```python
from build123d import *

# Parameters (mm, degrees)
SKETCH1_W           = 25
SKETCH1_H           = 21
BOSS_EXTRUDE1_DEPTH = 5
BOSS_EXTRUDE2_DEPTH = 8


with BuildPart() as part:
    # Sketch1 → Boss-Extrude1 (new body)
    with BuildSketch(Plane(origin=(0, 0, 0), x_dir=(1, 0, 0), z_dir=(0, 1, 0))):
        Rectangle(SKETCH1_W, SKETCH1_H)
    extrude(amount=BOSS_EXTRUDE1_DEPTH)

    # Sketch2 → Boss-Extrude2 (add)
    with BuildSketch(Plane(origin=(12.5, 0, 0), x_dir=(0, 0, -1), z_dir=(1, 0, 0))):
        with BuildLine():
            Line((-7.5, 1), (-6.3, 1))
            Line((-6.3, 1), (6.3, 4))
            Line((6.3, 4), (-7.5, 4))
            ThreePointArc((-7.5, 4), (-8.207106781, 3.707106781), (-8.5, 3))
            Line((-8.5, 3), (-8.5, 2))
            ThreePointArc((-8.5, 2), (-8.207106781, 1.292893219), (-7.5, 1))
        make_face()
        with BuildLine():
            Line((6.3, 4), (-6.3, 1))
            Line((-6.3, 1), (7.5, 1))
            ThreePointArc((7.5, 1), (8.207106781, 1.292893219), (8.5, 2))
            Line((8.5, 2), (8.5, 3))
            ThreePointArc((8.5, 3), (8.207106781, 3.707106781), (7.5, 4))
            Line((7.5, 4), (6.3, 4))
        make_face()
    extrude(amount=BOSS_EXTRUDE2_DEPTH)


solid = part.part
```
Source: CAD feature listing. Evaluate the final solid. Frame: model axes, mm. A direction names the side the tool comes from. Coordinates: 2 decimals unless noted, no trailing zeros. Loops run counter-clockwise (first coordinate to the right, second up) from the corner with the lowest first, then second, coordinate; pieces in that order, holes last. Notation, with made-up numbers: M 14.25,34.5 L 54.25,34.5 A16 cw 54.25,39.5 Z; hole C -19.75,-1 d7. An arc over 180 degrees is marked long. Use a Markdown table: item, result. Add a question column.
Q1. Access query for faces 1 (the cylindrical face through (16.444, 3.699, -8.215)), 2 (the cylindrical face through (16.444, 1.301, 8.215)), 3 (the flat face through (16.4, 2.5, -8.5)), 4 (the flat face through (16, 4, 0)). Directions: +Z, -Z, +X, -X, +Y, -Y. A direction counts if a zero-diameter tool reaches every point of the face in a straight line with its end or side. Return the directions, or none.
Q2. Section query C-C, the plane z = -9. Return loops of the section in (x, y).
Q3. Material intervals for L1, parallel to Y at x = 18, z = -0.5; L2, parallel to Z at x = 17.5, y = 2.1; L3, parallel to X at y = 4.5, z = 3.5, sorted ascending.
Q4. Section query A-A, the plane x = 14.5. Return loops of the section in (y, z).
Q5. Section query B-B, the plane z = 5.5. Return loops of the section in (x, y).
Q6. First-contact query: pin 1 (0.8 mm diameter, centred on x = 16.5, y = 2.5, fed in from -Z); pin 2 (6.5 mm diameter, centred on x = 17, z = 1, fed in from -Y); pin 3 (0.8 mm diameter, centred on x = 16.5, y = 2.5, fed in from +Z). Flat tips, straight axial feed; report the tip coordinate or a pass-through.
Result:
| question | item | result |
|---|---|---|
| 1 | face 1 | -Z, +X, +Y |
| 1 | face 2 | +Z, +X, -Y |
| 1 | face 3 | -Z, +X, +Y, -Y |
| 1 | face 4 | +Z, -Z, +X, +Y |
| 2 | outline | M -12.5,0 L 12.5,0 L 12.5,5 L -12.5,5 Z |
| 3 | L1 | y = 1 to 4 |
| 3 | L2 | z = -8.5 to 8.5 |
| 3 | L3 | x = -12.5 to 12.5 |
| 4 | outline | M 1,-7.5 A1 ccw 2,-8.5 L 3,-8.5 A1 ccw 4,-7.5 L 4,7.5 A1 ccw 3,8.5 L 2,8.5 A1 ccw 1,7.5 Z |
| 5 | outline | M -12.5,0 L 12.5,0 L 12.5,1 L 20.5,1 L 20.5,4 L 12.5,4 L 12.5,5 L -12.5,5 Z |
| 6 | pin 1 | stops at z = -8.5 |
| 6 | pin 2 | stops at y = 1 |
| 6 | pin 3 | stops at z = 8.5 |
